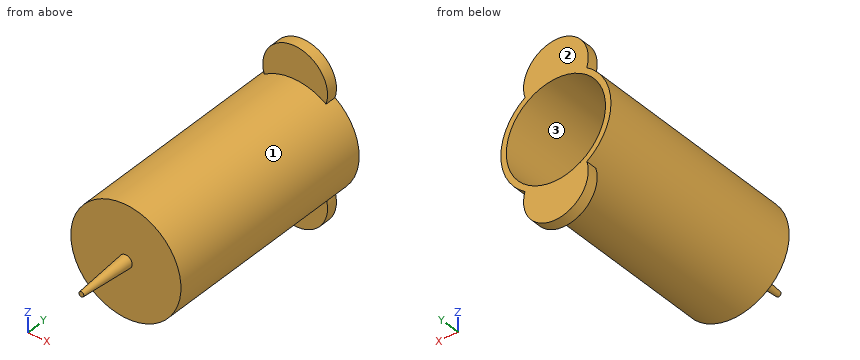
Autodesk Inventor part; units mm, degrees
ref_plane "YZ Plane" through (0, 0, 0) normal (1, 0, 0) x (0, 1, 0)
ref_plane "XZ Plane" through (0, 0, 0) normal (0, 1, 0) x (-1, 0, 0)
ref_plane "XY Plane" through (0, 0, 0) normal (0, 0, 1) x (1, 0, 0)
sketch "Sketch1" plane through (0, 0, 0) normal (0, 1, 0) x (-1, 0, 0)
  circle A0 centre (0, 0) radius 25.4
  dimension "d0" = 50.8
extrude "Extrusion1" add sketch "Sketch1" along normal blind 101.6
sketch "Sketch2" plane through (0, 101.6, 0) normal (0, 1, 0) x (1, 0, 0)
  circle A0 centre (0, 0) radius 25.4
  circle A1 centre (0, -25.4) radius 14.9225
  circle A2 centre (0, 25.4) radius 14.9225
  dimension "d3" = 29.845
  dimension "d4" = 29.845
extrude "Extrusion2" add sketch "Sketch2" against normal blind 5.08
sketch "Sketch3" plane through (0, 101.6, 0) normal (0, 1, 0) x (1, 0, 0)
  circle A0 centre (0, 0) radius 22.86
  dimension "d7" = 45.72
extrude "Extrusion3" cut sketch "Sketch3" against normal blind 195.072
sketch "Sketch4" plane through (0, 0, 0) normal (0, -1, 0) x (1, 0, 0)
  circle A0 centre (0, 0) radius 2.921
  dimension "d10" = 5.842
extrude "Extrusion4" add sketch "Sketch4" along normal blind 25.4 draft -4
sketch "Sketch5" plane through (0, 0, 0) normal (0, -1, 0) x (1, 0, 0)
  circle A0 centre (0, 0) radius 1.1449
  circle A1 centre (0, 0) radius 22.86
extrude "Extrusion5" add sketch "Sketch5" against normal blind 2.54
properties part number "ReducedLargeSyrgine"
Read the model definition and answer for the solid it produces. Units are mm, in the model's axes. Face numbers are marked on the shaded views. Round coordinates to 2 decimals unless told otherwise and drop trailing zeros. Write each loop counter-clockwise with the first axis right and the second up, starting at its lowest first coordinate (ties: lowest second). Pieces come first, ordered by that corner, then holes. Notation, with made-up numbers: (-18.75, 18.5) - (25.25, 18.5) arc R24 cw to (25.25, 40.5) - close; hole circle Ø4 at (33.5, 81). An arc over 180 degrees is marked (long way). One line per question, with ' | ' between items. Start each with the question number.
1. Section B-B (y = 44) is taken. Determine the outline of the cut face in (x, z).
2. Each of these flat-tipped pins is pushed along its axis until it touches: pin 1 (8 mm diameter, centred on x = 9.5, y = 47.5, fed in from -Z); pin 2 (5 mm diameter, centred on x = -11, z = -13.5, fed in from -Y); pin 3 (1.5 mm diameter, centred on y = 25.5, z = 11.5, fed in from -X). Where does it stop, or does it pass through?
3. For a pull along X with two mould halves and no side action, classify the marked faces 1, 2 and 3 as +X half, -X half, draft (parallel to the pull), parting line (faces both ways), or undercut.
4. Section D-D (x = 6) is taken. Determine the outline of the cut face in (y, z), and give its area (3 significant figures).
5. Section A-A (z = -7) is taken. Determine the outline of the cut face in (x, y).
6. Section C-C (x = -8) is taken. Determine the outline of the cut face in (y, z).
7. Find the intervals of material crossed by probe 1 along Z at (x, y) = (0, 73); probe 2 along Z at (x, y) = (0, 1); probe 3 along Y at (x, z) = (-3, -24), in increasing order. Write a range as [from, to].
Filled in:
1) outline: circle Ø50.8 at (0, 0); hole circle Ø45.72 at (0, 0)
2) pin 1: z = -24.8 | pin 2: y = 0 | pin 3: x = -23.01
3) face 1: parting line | face 2: draft | face 3: undercut
4) outline: (0, -24.68) - (96.52, -24.68) - (96.52, -39.06) - (101.6, -39.06) - (101.6, -22.06) - (2.54, -22.06) - (2.54, 22.06) - (101.6, 22.06) - (101.6, 39.06) - (96.52, 39.06) - (96.52, 24.68) - (0, 24.68) - close | area: 791 mm²
5) outline: (-24.42, 0) - (24.42, 0) - (24.42, 101.6) - (21.76, 101.6) - (21.76, 2.54) - (-21.76, 2.54) - (-21.76, 101.6) - (-24.42, 101.6) - close
6) outline: (0, -24.11) - (96.52, -24.11) - (96.52, -38) - (101.6, -38) - (101.6, -21.41) - (2.54, -21.41) - (2.54, 21.41) - (101.6, 21.41) - (101.6, 38) - (96.52, 38) - (96.52, 24.11) - (0, 24.11) - close
7) probe 1: [-25.4, -22.86], [22.86, 25.4] | probe 2: [-25.4, -1.14], [1.14, 25.4] | probe 3: [0, 101.6]
